```python
from build123d import *

# Parameters (mm, degrees)
BOSS_EXTRUDE1_DEPTH = 3.175
SKETCH2_R           = 1.5875
SKETCH2_W           = 80.264
SKETCH2_H           = 12.954
CUT_EXTRUDE1_DEPTH  = 223.985606318
SKETCH7_R           = 1.5875
SKETCH7_W           = 46.99
SKETCH7_H           = 138.43
CUT_EXTRUDE4_DEPTH  = 223.985606318
CUT_EXTRUDE5_DEPTH  = 223.985606318
CUT_EXTRUDE6_DEPTH  = 221.482742149
CUT_EXTRUDE7_DEPTH  = 221.482742149


with BuildPart() as part:
    # Sketch1 → Boss-Extrude1 (new body)
    with BuildSketch(Plane(origin=(0, 0, 0), x_dir=(1, 0, 0), z_dir=(0, 1, 0))):
        with BuildLine():
            Line((-80, 112.5), (100, 112.5))
            Line((100, 112.5), (100, -112.5))
            Line((100, -112.5), (-80, -112.5))
            ThreePointArc((-80, -112.5), (-192.5, 0), (-80, 112.5))
        make_face()
    extrude(amount=-BOSS_EXTRUDE1_DEPTH)

    # Sketch2 → Cut-Extrude1 (cut, through all)
    with BuildSketch(Plane(origin=(0, 0, 0), x_dir=(1, 0, 0), z_dir=(0, 1, 0))):
        with Locations(Location((36.144045702, -74.2188, 0), (0, 0, 270))):
            Circle(SKETCH2_R)
        with Locations(Location((36.144045702, -67.8688, 0), (0, 0, 270))):
            Circle(SKETCH2_R)
        with Locations(Location((36.144045702, -61.5188, 0), (0, 0, 270))):
            Circle(SKETCH2_R)
        with Locations(Location((36.144045702, -55.1688, 0), (0, 0, 270))):
            Circle(SKETCH2_R)
        with Locations(Location((36.144045702, -48.8188, 0), (0, 0, 270))):
            Circle(SKETCH2_R)
        with Locations(Location((36.144045702, -42.4688, 0), (0, 0, 270))):
            Circle(SKETCH2_R)
        with Locations(Location((36.144045702, -36.1188, 0), (0, 0, 270))):
            Circle(SKETCH2_R)
        with Locations(Location((67.894045702, -74.2188, 0), (0, 0, 270))):
            Circle(SKETCH2_R)
        with Locations(Location((67.894045702, -67.8688, 0), (0, 0, 270))):
            Circle(SKETCH2_R)
        with Locations(Location((67.894045702, -61.5188, 0), (0, 0, 270))):
            Circle(SKETCH2_R)
        with Locations(Location((67.894045702, -55.1688, 0), (0, 0, 270))):
            Circle(SKETCH2_R)
        with Locations(Location((67.894045702, -48.8188, 0), (0, 0, 270))):
            Circle(SKETCH2_R)
        with Locations(Location((67.894045702, -42.4688, 0), (0, 0, 270))):
            Circle(SKETCH2_R)
        with Locations(Location((67.894045702, -36.1188, 0), (0, 0, 270))):
            Circle(SKETCH2_R)
        with Locations(Location((36.144045702, 74.2188, 0), (0, 0, 270))):
            Circle(SKETCH2_R)
        with Locations(Location((36.144045702, 67.8688, 0), (0, 0, 270))):
            Circle(SKETCH2_R)
        with Locations(Location((36.144045702, 61.5188, 0), (0, 0, 270))):
            Circle(SKETCH2_R)
        with Locations(Location((36.144045702, 55.1688, 0), (0, 0, 270))):
            Circle(SKETCH2_R)
        with Locations(Location((36.144045702, 48.8188, 0), (0, 0, 270))):
            Circle(SKETCH2_R)
        with Locations(Location((36.144045702, 42.4688, 0), (0, 0, 270))):
            Circle(SKETCH2_R)
        with Locations(Location((36.144045702, 36.1188, 0), (0, 0, 270))):
            Circle(SKETCH2_R)
        with Locations(Location((67.894045702, 74.2188, 0), (0, 0, 270))):
            Circle(SKETCH2_R)
        with Locations(Location((67.894045702, 67.8688, 0), (0, 0, 270))):
            Circle(SKETCH2_R)
        with Locations(Location((67.894045702, 61.5188, 0), (0, 0, 270))):
            Circle(SKETCH2_R)
        with Locations(Location((67.894045702, 55.1688, 0), (0, 0, 270))):
            Circle(SKETCH2_R)
        with Locations(Location((67.894045702, 48.8188, 0), (0, 0, 270))):
            Circle(SKETCH2_R)
        with Locations(Location((67.894045702, 42.4688, 0), (0, 0, 270))):
            Circle(SKETCH2_R)
        with Locations(Location((67.894045702, 36.1188, 0), (0, 0, 270))):
            Circle(SKETCH2_R)
        with Locations((52.019045702, -96.4438)):
            Rectangle(SKETCH2_W, SKETCH2_H)
        with Locations((52.019045702, 96.4438)):
            Rectangle(SKETCH2_W, SKETCH2_H)
    extrude(amount=-CUT_EXTRUDE1_DEPTH, mode=Mode.SUBTRACT)

    # Sketch7 → Cut-Extrude4 (cut, through all)
    with BuildSketch(Plane(origin=(0, 0, 0), x_dir=(1, 0, 0), z_dir=(0, 1, 0))):
        with Locations(Location((-50.166143469, 0, 0), (0, 0, 270))):
            Circle(SKETCH7_R)
        with Locations(Location((25.582761582, 0, 0), (0, 0, 270))):
            Circle(SKETCH7_R)
        with Locations(Location((87.462148806, 0, 0), (0, 0, 270))):
            Circle(SKETCH7_R)
        with Locations((-13.971143469, 0)):
            Rectangle(SKETCH7_W, SKETCH7_H)
    extrude(amount=-CUT_EXTRUDE4_DEPTH, mode=Mode.SUBTRACT)

    # Sketch8 → Cut-Extrude5 (cut, through all)
    with BuildSketch(Plane(origin=(0, 0, 0), x_dir=(1, 0, 0), z_dir=(0, 1, 0))):
        with BuildLine():
            Line((-167.0966, 25.4), (-229.776686608, 25.4))
            Line((-229.776686608, 25.4), (-229.776686608, -25.4))
            Line((-229.776686608, -25.4), (-167.0966, -25.4))
            ThreePointArc((-167.0966, -25.4), (-141.6966, 0), (-167.0966, 25.4))
        make_face()
    extrude(amount=-CUT_EXTRUDE5_DEPTH, mode=Mode.SUBTRACT)

    # Sketch9 → Cut-Extrude6 (cut, through all)
    with BuildSketch(Plane(origin=(0, 0, 0), x_dir=(1, 0, 0), z_dir=(0, 1, 0))):
        Polygon((0, 120.924498436), (0, 78.840642152), (20.45905334, 78.840642152), (20.45905334, -78.840642152), (0, -78.840642152), (0, -122.522619561), (114.748199697, -122.522619561), (114.748199697, 120.924498436), align=None)
    extrude(amount=-CUT_EXTRUDE6_DEPTH, mode=Mode.SUBTRACT)

    # Sketch10 → Cut-Extrude7 (cut, through all)
    with BuildSketch(Plane(origin=(0, 0, 0), x_dir=(1, 0, 0), z_dir=(0, 1, 0))):
        Polygon((24.720709672, 75.644399903), (-63.708659228, 75.644399903), (-63.708659228, -78.30793511), (24.720709672, -78.30793511), (24.720709672, -86.831247776), (24.720709672, -123.055326602), (-234.174912529, -128.382397018), (-239.283531036, 119.896462399), (24.720709672, 119.896462399), align=None)
    extrude(amount=-CUT_EXTRUDE7_DEPTH, mode=Mode.SUBTRACT)


solid = part.part
```
The listing builds one solid part. Answer for the finished solid, in the listing's coordinates (mm). A direction names the side the tool comes from. Round coordinates to 2 decimals unless told otherwise and drop trailing zeros. Loops run counter-clockwise (first coordinate to the right, second up) from the corner with the lowest first, then second, coordinate; pieces in that order, holes last. Notation, with made-up numbers: (-18, 58.25) -> (-6, 58.25) arc R14 cw to (-6, 75.25) -> close; hole circle Ø8 at (79, 73). An arc over 180 degrees is marked (long way). Use one line per item in the form item = value.
1. The part is cut by section B-B on x = -0.5. Determine the outline of the cut face in (y, z) (3 decimals), and give its area (3 significant figures).
Answer key:
outline = (-3.175, -75.644) -> (0, -75.644) -> (0, -69.215) -> (-3.175, -69.215) -> close; (-3.175, 69.215) -> (0, 69.215) -> (0, 78.308) -> (-3.175, 78.308) -> close
area = 49.3 mm²
2. The part is cut by section C-C on y = -1.3. Determine the outline of the cut face in (x, z) (1 decimal).
Answer key:
outline = (-63.7, -75.6) -> (20.5, -75.6) -> (20.5, 78.3) -> (-63.7, 78.3) -> close; hole circle Ø3.2 at (-50.2, 0); hole (-37.5, -69.2) -> (9.5, -69.2) -> (9.5, 69.2) -> (-37.5, 69.2) -> close
3. The part is cut by section A-A on z = 12. Determine the outline of the cut face in (x, y) (3 decimals), and give its area (3 significant figures).
Answer key:
outline = (-63.709, -3.175) -> (-37.466, -3.175) -> (-37.466, 0) -> (-63.709, 0) -> close; (9.524, -3.175) -> (20.459, -3.175) -> (20.459, 0) -> (9.524, 0) -> close
area = 118 mm²
4. A tool of negligible diameter and unlimited length cuts with its end or side. For faces 5 (the flat face through (9.524, -2, 1)), 6 (the flat face through (-40, 0, 0)), from which of +Z, -Z, +X, -X, +Y, -Y can it reach the whole face along a straight path? Write none if from no direction.
Answer key:
face_5 = +Y, -Y
face_6 = +Z, -Z, +X, -X, +Y
5. Find the intervals of material crossed by probe 1 along X at (y, z) = (-1.1, 0); probe 2 along Z at (x, y) = (-32.5, -1.6) (3 decimals); probe 3 along X at (y, z) = (-1.55, -35.5), in increasing order. Write a range as [from, to].
Answer key:
probe_1 = [-63.71, -51.75], [-48.58, -37.47], [9.52, 20.46]
probe_2 = [-75.644, -69.215], [69.215, 78.308]
probe_3 = [-63.71, -37.47], [9.52, 20.46]
6. For a pull along Z with two mould halves and no side action, classify faces 1 (the flat face through (-40, -3.175, 0)), 2 (the flat face through (-22, -2, 78.308)), 3 (the flat face through (-14, -2, -69.215)), 4 (the flat face through (-37.466, -2, 1)) as released by +Z, released by -Z, zero draft, split by the parting line, or undercut.
Answer key:
face_1 = zero draft
face_2 = released by +Z
face_3 = undercut
face_4 = undercut
